```python
from build123d import *

# Parameters (mm, degrees)
SKETCH2_W           = 29
SKETCH2_H           = 30
SKETCH2_W_2         = 5.4
SKETCH2_H_2         = 3.5
SKETCH2_W_3         = 5.8
SKETCH2_H_3         = 5.3
BOSS_EXTRUDE1_DEPTH = 13
CUT_EXTRUDE1_DEPTH  = 5.3


with BuildPart() as part:
    # Sketch2 → Boss-Extrude1 (new body)
    with BuildSketch(Plane(origin=(0, 0, 0), x_dir=(0, 0, -1), z_dir=(1, 0, 0))):
        Rectangle(SKETCH2_W, SKETCH2_H)
        with Locations((-17.2, 5.55)):
            Rectangle(SKETCH2_W_2, SKETCH2_H_2)
        with Locations((4.1, 17.65)):
            Rectangle(SKETCH2_W_3, SKETCH2_H_3)
        with Locations((17.2, 5.55)):
            Rectangle(SKETCH2_W_2, SKETCH2_H_2)
    extrude(amount=BOSS_EXTRUDE1_DEPTH)

    # Sketch3 → Cut-Extrude1 (cut)
    with BuildSketch(Plane(origin=(0, 15, 0), x_dir=(1, 0, 0), z_dir=(0, 1, 0))):
        with BuildLine():
            Line((6.5, 1.2), (9.4, 1.2))
            Line((9.4, 1.2), (9.4, 4.1))
            ThreePointArc((9.4, 4.1), (8.550609665, 2.049390335), (6.5, 1.2))
        make_face()
        with BuildLine():
            ThreePointArc((6.5, 7), (8.550609665, 6.150609665), (9.4, 4.1))
            Line((9.4, 4.1), (9.4, 7))
            Line((9.4, 7), (6.5, 7))
        make_face()
        with BuildLine():
            ThreePointArc((3.6, 4.1), (4.449390335, 6.150609665), (6.5, 7))
            Line((6.5, 7), (3.6, 7))
            Line((3.6, 7), (3.6, 4.1))
        make_face()
        with BuildLine():
            Line((3.6, 1.2), (6.5, 1.2))
            ThreePointArc((6.5, 1.2), (4.449390335, 2.049390335), (3.6, 4.1))
            Line((3.6, 4.1), (3.6, 1.2))
        make_face()
        Polygon((0, 1.2), (3.6, 1.2), (3.6, 4.1), (3.6, 7), (0, 7), align=None)
        Polygon((9.4, 1.2), (13, 1.2), (13, 7), (9.4, 7), (9.4, 4.1), align=None)
    extrude(amount=CUT_EXTRUDE1_DEPTH, mode=Mode.SUBTRACT)


solid = part.part
```
Verification items for the finished model (mm, model axes). A direction names the side the tool comes from. Coordinates: 2 decimals unless noted, no trailing zeros. Write each loop counter-clockwise with the first axis right and the second up, starting at its lowest first coordinate (ties: lowest second). Pieces come first, ordered by that corner, then holes. Notation, with made-up numbers: M 8,2 L 54,2 A12 ccw 54,16 Z; hole C 24.5,76 d5. An arc over 180 degrees is marked long. Answer as a JSON object with one key per item and string values. Group by question number.
(1) Tool access check on faces 1 (the face through (6, 3.8, -17)), 2 (the face through (6, 7.3, -17)), 3 (the face through (6, 7.3, 17)), 4 (the face through (6, -6, 14.5)). Record the directions out of +Z, -Z, +X, -X, +Y, -Y that give a thin tool (end or side, any length) a straight path to the whole face; none if there is none.
(2) Cross-section at B-B, the plane z = -15.5. Record the cut outline in (x, y), and give its area (3 significant figures).
(3) Cross-section at C-C, the plane y = -6. Record the cut outline in (x, z), and give its area (3 significant figures).
(4) Cross-section at D-D, the plane x = 8.5. Record the cut outline in (y, z), and give its area (3 significant figures).
(5) Material ranges on line 1 (Z direction, x = 5.5, y = -9.5); line 2 (Y direction, x = 5, z = -14); line 3 (Y direction, x = 3, z = -15), recorded low to high.
(6) Gauge pin test, flat ends, axial feed: pin 1 (6.5 mm diameter, centred on x = 8.5, y = -1.5, fed in from -Z); pin 2 (4.5 mm diameter, centred on x = 8, z = 18.5, fed in from +Y); pin 3 (4.5 mm diameter, centred on x = 4.5, z = 18, fed in from -Y). Record the tip position at first contact, or that the pin passes through.
(7) Cross-section at A-A, the plane x = 1.25. Record the cut outline in (y, z), and give its area (3 significant figures).
Reply:
{
 "1": {"face 1": "-Z, +X, -X, -Y", "face 2": "-Z, +X, -X, +Y", "face 3": "+Z, +X, -X, +Y", "face 4": "+Z, +X, -X, -Y"},
 "2": {"outline": "M 0,3.8 L 13,3.8 L 13,7.3 L 0,7.3 Z", "area": "45.5 mm²"},
 "3": {"outline": "M 0,-14.5 L 13,-14.5 L 13,14.5 L 0,14.5 Z", "area": "377 mm²"},
 "4": {"outline": "M -15,-14.5 L 3.8,-14.5 L 3.8,-19.9 L 7.3,-19.9 L 7.3,-14.5 L 15,-14.5 L 15,-6.2 L 20.3,-6.2 L 20.3,-2 L 15,-2 L 15,14.5 L 7.3,14.5 L 7.3,19.9 L 3.8,19.9 L 3.8,14.5 L -15,14.5 Z", "area": "930 mm²"},
 "5": {"line 1": "-14.5 to 14.5", "line 2": "-15 to 15", "line 3": "3.8 to 7.3"},
 "6": {"pin 1": "z = -14.5", "pin 2": "y = 7.3", "pin 3": "y = 3.8"},
 "7": {"outline": "M -15,-14.5 L 3.8,-14.5 L 3.8,-19.9 L 7.3,-19.9 L 7.3,-14.5 L 15,-14.5 L 15,14.5 L 7.3,14.5 L 7.3,19.9 L 3.8,19.9 L 3.8,14.5 L -15,14.5 Z", "area": "908 mm²"}
}
